Verification items for the finished model (mm, model axes). Face numbers are marked on the shaded views. Give positions to 0.01 mm unless a question says otherwise; leave off trailing zeros. Write each loop counter-clockwise with the first axis right and the second up, starting at its lowest first coordinate (ties: lowest second). Pieces come first, ordered by that corner, then holes. Notation, with made-up numbers: (1, 13.5) -> (38, 13.5) arc R14 ccw to (38, 35.5) -> close; hole circle Ø6 at (29, -27.75). An arc over 180 degrees is marked (long way). Answer as CSV lines item,"result". Start each with the question number.
1) Material ranges on L1, parallel to X at y = -67.5, z = 1.9; L2, parallel to Y at x = -81.5, z = 1.85; L3, parallel to X at y = 81, z = 1.7, recorded low to high.
2) Sectioned sample at A-A on x = -139. Record the cut outline in (y, z).
3) Gauge pin test, flat end, axial feed: pin 1 Ø1.5 at (x, y) = (-94.5, -67.5) entering from +Z. Record the tip position at first contact, or that the pin passes through.
4) Mould release check, pull along Z, two halves, no side actions. Record for the marked faces 1 and 2: released by +Z, released by -Z, zero draft, split by the parting line, or undercut.
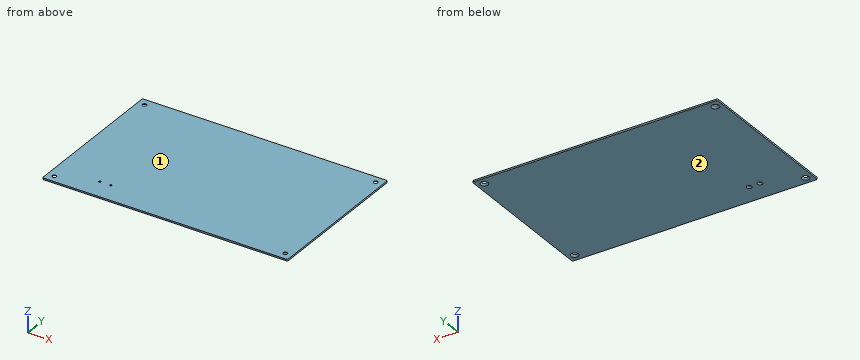
```python
from build123d import *

# Parameters (mm, degrees)
BASE_FLANGE1_DEPTH             = 2
FURO_ROSCADO_DE_M31_AT_2_COUNT = 2
FURO_ROSCADO_DE_M31_AT_2_PITCH = 13


# Sheet-metal steps are written as plain solids
with BuildPart() as part:
    # Sketch1 → Base-Flange1 (new body)
    with BuildSketch(Plane.XY):
        with BuildLine():
            Line((-146, 92.5), (146, 92.5))
            ThreePointArc((146, 92.5), (147.060660172, 92.060660172), (147.5, 91))
            Line((147.5, 91), (147.5, -91))
            ThreePointArc((147.5, -91), (147.060660172, -92.060660172), (146, -92.5))
            Line((146, -92.5), (-146, -92.5))
            ThreePointArc((-146, -92.5), (-147.060660172, -92.060660172), (-147.5, -91))
            Line((-147.5, -91), (-147.5, 91))
            ThreePointArc((-147.5, 91), (-147.060660172, 92.060660172), (-146, 92.5))
        make_face()
    extrude(amount=BASE_FLANGE1_DEPTH)

    # Esboço3 → Furo roscado de M41 (revolve, cut)
    with BuildSketch(Plane(origin=(-139, 83.5, 2), x_dir=(0, -1, 0), z_dir=(1, 0, 0))):
        Polygon((0, 0), (0, 2), (4.5, 2), (1.65, -0.85), (1.65, 0), align=None)
    furo_roscado_de_m41 = revolve(axis=Axis((-139, 83.5, 8.35), (0, 0, -1)), mode=Mode.SUBTRACT)

    # Espelhar1: Furo roscado de M41 across plane
    add(furo_roscado_de_m41.mirror(Plane.ZX), mode=Mode.SUBTRACT)

    # Espelhar2: Furo roscado de M41 across plane
    add(furo_roscado_de_m41.mirror(Plane(origin=(0, 0, 0), x_dir=(0, 0, 1), z_dir=(1, 0, 0))), mode=Mode.SUBTRACT)

    # Espelhar2 copy 1 sketch → Espelhar2 copy 1 (revolve, cut)
    with BuildSketch(Plane(origin=(139, -83.5, 2), x_dir=(0, 1, 0), z_dir=(-1, 0, 0))):
        Polygon((0, 0), (0, 2), (4.5, 2), (1.65, -0.85), (1.65, 0), align=None)
    revolve(axis=Axis((139, -83.5, 8.35), (0, 0, -1)), mode=Mode.SUBTRACT)

    # Esboço5 → Furo roscado de M31 (revolve, cut)
    with BuildSketch(Plane(origin=(-94.5, -67.5, 2), x_dir=(0, -1, 0), z_dir=(1, 0, 0))):
        Polygon((0, 0), (0, 2), (3, 2), (1.25, 0.25), (1.25, 0), align=None)
    furo_roscado_de_m31 = revolve(axis=Axis((-94.5, -67.5, 8.35), (0, 0, -1)), mode=Mode.SUBTRACT)

    # Furo roscado de M31 at 2: Furo roscado de M31 ×2
    with Locations(*[(i * FURO_ROSCADO_DE_M31_AT_2_PITCH, 0, 0) for i in range(1, FURO_ROSCADO_DE_M31_AT_2_COUNT)]):
        add(furo_roscado_de_m31, mode=Mode.SUBTRACT)


solid = part.part
```
Ans:
1,L1,"x = -147.5 to -95.75, -93.25 to -82.75, -80.25 to 147.5"
1,L2,"y = -92.5 to -68.75, -66.25 to 92.5"
1,L3,"x = -147.5 to -140.26, -137.74 to 137.74, 140.26 to 147.5"
2,outline,"(-92.5, 0) -> (-88, 0) -> (-86, 2) -> (-92.5, 2) -> close; (-81, 2) -> (-79, 0) -> (79, 0) -> (81, 2) -> close; (86, 2) -> (88, 0) -> (92.5, 0) -> (92.5, 2) -> close"
3,pin 1,"passes through"
4,face 1,"released by +Z"
4,face 2,"released by -Z"
